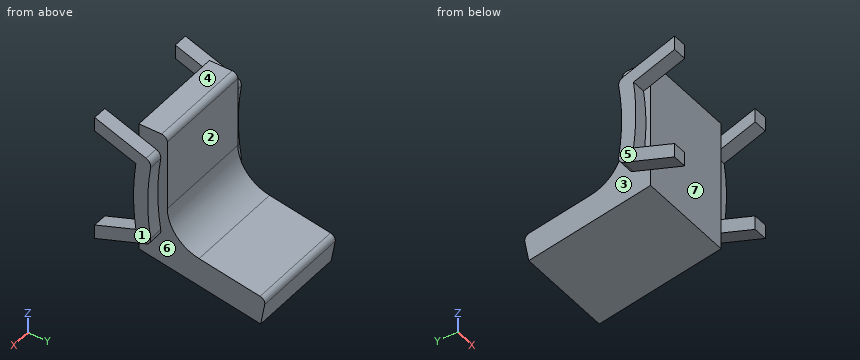
Autodesk Inventor part; units mm, degrees
ref_plane "Plano de trabajo1" through (-35, 0, 0) normal (1, 0, 0) x (0, 0, -1)
ref_plane "YZ Plane" through (0, 0, 0) normal (1, 0, 0) x (0, 1, 0)
ref_plane "XZ Plane" through (0, 0, 0) normal (0, 1, 0) x (-1, 0, 0)
sketch "Boceto1" plane through (0, 0, 0) normal (1, 0, 0) x (0, 1, 0)
  line L0 (85.212, 5.2834) -> (42.3115, 12.8479)
  arc A0 (20, 39.4377) -> (42.3115, 12.8479) centre (47, 39.4377) ccw
  line L1 (20, 39.4377) -> (20, 89)
  line L2 (16, 93) -> (0, 93)
  line L3 (0, 93) -> (0, 0)
  line L4 (0, 0) -> (85.6783, -15.1074)
  line L5 (85.6783, -15.1074) -> (88.4566, 0.6495)
  arc A1 (88.4566, 0.6495) -> (85.212, 5.2834) centre (84.5174, 1.3441) ccw
  arc A2 (20, 89) -> (16, 93) centre (16, 89) ccw
  line L6 (-24, 93) -> (12.0957, 79.8622)
  line L7 (12.0957, 16.1378) -> (-24, 3)
  line L8 (-24, 3) -> (-24, 13)
  line L9 (-24, 13) -> (4.9435, 23.5346)
  line L10 (4.9435, 72.4654) -> (-24, 83)
  line L11 (-24, 83) -> (-24, 93)
  arc A3 (15.327, 74.4007) -> (15.327, 21.5993) centre (186.3007, 48) ccw
  arc A4 (4.9435, 72.4654) -> (4.9435, 23.5346) centre (186.3007, 48) ccw
  arc A5 (15.327, 74.4007) -> (12.0957, 79.8622) centre (10.3856, 75.1638) ccw
  arc A6 (12.0957, 16.1378) -> (15.327, 21.5993) centre (10.3856, 20.8362) ccw
  point P0 (20, 93)
  point P1 (89.1512, 4.5888)
  point P2 (16, 78.4412)
  point P3 (16, 17.5588)
  dimension "d0" = 87
  dimension "d1" = 20
  dimension "d2" = 20
  dimension "d3" = 27
  dimension "d4" = 100
  dimension "d5" = 93
  dimension "d6" = 4
  dimension "d7" = 24
  dimension "d8" = 16
  dimension "d9" = 110
  dimension "d10" = 90
  dimension "d11" = 70
  dimension "d12" = 10
  dimension "d13" = 10
  dimension "d14" = 3
  dimension "d17" = 110
  dimension "d23" = 173
  dimension "d24" = 10
  dimension "d25" = 183
  dimension "d26" = 5
extrude "Extrusión1" add sketch "Boceto1" against normal blind 70 contours A1 L5 L4 L3 L7 A6 A3 A5 L6 L2 A2 L1 A0 L0 | L3 L9 A4 L10 L6 A5 A3 A6 L7 | L3 L10 A4 L9
extrude "Extrusión2" add sketch "Boceto1" along normal blind 10 contours L7 L8 L9 L3 | L3 L9 A4 L10 L6 A5 A3 A6 L7 | L3 L10 L11 L6
ref_plane "Plano de trabajo1" through (-35, 0, 0) normal (1, 0, 0) x (0, 0, -1)
mirror "Simetría1" about plane through (-35, 0, 0) normal (1, 0, 0) of "Extrusión2"
properties part number "Pieza de practica 14"
The model under review builds one solid part; all positions refer to its coordinate system, in mm. Face numbers are marked on the shaded views. A direction names the side the tool comes from. Round coordinates to 2 decimals unless told otherwise and drop trailing zeros. Loops run counter-clockwise (first coordinate to the right, second up) from the corner with the lowest first, then second, coordinate; pieces in that order, holes last. Notation, with made-up numbers: (47.25, 41.25) - (75.25, 41.25) arc R35 cw to (75.25, 76.25) - close; hole circle Ø5 at (69, 75.25). An arc over 180 degrees is marked (long way). Use a Markdown table: item, result. Add a question column.
Q1. For probe 1 along X at (y, z) = (-18, 81); probe 2 along Y at (x, z) = (-25, 64); probe 3 along X at (y, z) = (60, 7), list the stretches that pass through material, from the lowest coordinate up.
Q2. Insertion check: pin 1 Ø21 at (x, z) = (-33, 39.5) entering from -Y; pin 2 Ø1.5 at (y, z) = (2.5, 37.5) entering from +X; pin 3 Ø2 at (x, y) = (-48, 22) entering from -Z. Each pin has a flat end and moves straight along its axis. Give the tip position at first contact, or say it passes through.
Q3. Machinability: for the marked faces 1, 2 and 3, which of the approach directions +Z, -Z, +X, -X, +Y, -Y give a long, thin tool a straight path to every point of the face, cutting with its end or side? Answer none if there is none.
Q4. The part is to be moulded in two halves that separate along X. For the marked faces 4, 5, 6 and 7, say which applies: pulls with the +X half, pulls with the -X half, needs draft (parallel to the pull), parting line crosses it, or undercut.
Q5. Add section C-C (y = 27.5). State the section outline as (x, z) points, plus the area to 3 significant figures.
Q6. Add section D-D (y = 45). State the section outline as (x, z) points.
Q7. Add section A-A (x = -47.5). State the section outline as (y, z) points, plus the area to 3 significant figures.
Q8. Add section B-B (z = 77.5). State the section outline as (x, y) points, plus the area to 3 significant figures.
Worked answers:
| question | item | result |
|---|---|---|
| 1 | probe 1 | -80 to -70, 0 to 10 |
| 1 | probe 2 | 0 to 20 |
| 1 | probe 3 | -70 to 0 |
| 2 | pin 1 | y = 0 |
| 2 | pin 2 | x = 0 |
| 2 | pin 3 | z = -4.06 |
| 3 | face 1 | +Z, -Z, +X, +Y, -Y |
| 3 | face 2 | +Z, +X, -X, +Y |
| 3 | face 3 | -X, +Y |
| 4 | face 4 | needs draft |
| 4 | face 5 | pulls with the -X half |
| 4 | face 6 | pulls with the +X half |
| 4 | face 7 | undercut |
| 5 | outline | (-70, -4.85) - (0, -4.85) - (0, 20.76) - (-70, 20.76) - close |
| 5 | area | 1,790 mm² |
| 6 | outline | (-70, -7.93) - (0, -7.93) - (0, 12.37) - (-70, 12.37) - close |
| 7 | outline | (0, 0) - (85.68, -15.11) - (88.46, 0.65) arc R4 ccw to (85.21, 5.28) - (42.31, 12.85) arc R27 cw to (20, 39.44) - (20, 89) arc R4 ccw to (16, 93) - (0, 93) - close |
| 7 | area | 3,360 mm² |
| 8 | outline | (-80, -8.89) - (-70, -8.89) - (-70, 0) - (0, 0) - (0, -8.89) - (10, -8.89) - (10, 14.81) - (0, 14.81) - (0, 20) - (-70, 20) - (-70, 14.81) - (-80, 14.81) - close |
| 8 | area | 1,870 mm² |
